Part model, mm, in its own coordinate system. A direction names the side the tool comes from. Round coordinates to 2 decimals unless told otherwise and drop trailing zeros. Loops run counter-clockwise (first coordinate to the right, second up) from the corner with the lowest first, then second, coordinate; pieces in that order, holes last. Notation, with made-up numbers: (-20.75, 76) - (24.25, 76) arc R24 cw to (24.25, 115) - close; hole circle Ø7 at (40, 48). An arc over 180 degrees is marked (long way). Put each result on its own line as item: value.
from build123d import *

# Parameters (mm, degrees)
SKETCH1_R           = 36
SKETCH1_R_2         = 13
BOSS_EXTRUDE1_DEPTH = 60
SKETCH2_W           = 9
SKETCH2_H           = 55


with BuildPart() as part:
    # Sketch1 → Boss-Extrude1 (new body)
    with BuildSketch(Plane(origin=(0, 0, 0), x_dir=(1, 0, 0), z_dir=(0, 1, 0))):
        Circle(SKETCH1_R)
        Circle(SKETCH1_R_2, mode=Mode.SUBTRACT)
    extrude(amount=BOSS_EXTRUDE1_DEPTH)

    # Sketch2 → Cut-Revolve1 (revolve, cut)
    with BuildSketch(Plane.XY):
        with Locations((-31.5, 30)):
            Rectangle(SKETCH2_W, SKETCH2_H)
    revolve(axis=Axis((0, 0, 0), (0, 1, 0)), mode=Mode.SUBTRACT)


solid = part.part
1. Band-saw the part on D-D (z = 23). List the corners of the cut face in (x, y).
A:
outline: (-27.69, 0) - (27.69, 0) - (27.69, 2.5) - (14.14, 2.5) - (14.14, 57.5) - (27.69, 57.5) - (27.69, 60) - (-27.69, 60) - (-27.69, 57.5) - (-14.14, 57.5) - (-14.14, 2.5) - (-27.69, 2.5) - close
2. Band-saw the part on C-C (y = 10). List the corners of the cut face in (x, z), plus the area to 3 significant figures.
A:
outline: circle Ø54 at (0, 0); hole circle Ø26 at (0, 0)
area: 1,760 mm²
3. Tool access for faces 1 (the flat face through (-5, 2.5, 27)), 2 (the cylindrical face through (-10.316, 29.58, 7.91)): list every direction of +Z, -Z, +X, -X, +Y, -Y with a clear straight run to the whole face (end or side of a thin tool).
A:
face 1: none
face 2: +Y, -Y
4. Two-plate mould, pull along Y, no slides. Class faces 3 (the flat face through (-1, 60, 15)), 4 (the flat face through (-5, 57.5, 27)), 5 (the cylindrical face through (-4.686, 1.232, -35.694)): pulls with the +Y half, pulls with the -Y half, needs draft (parallel to the pull), parting line crosses it, or undercut.
A:
face 3: pulls with the +Y half
face 4: undercut
face 5: needs draft
5. Pin check, flat tips, straight feed: P1, Ø12, axis at y = 45, z = -13.5, coming from the -X side; P2, Ø10, axis at x = -10.5, y = 43, coming from the -Z side; P3, Ø21.5, axis at x = 16.5, z = 10.5, coming from the -Y side; P4, Ø8, axis at y = 38, z = -13, coming from the -X side. Stop position of each tip, or through.
A:
P1: stops at x = -25.94
P2: stops at z = -26.43
P3: stops at y = 0
P4: stops at x = -25.46
6. Band-saw the part on B-B (z = 0). List the corners of the cut face in (x, y), plus the area to 3 significant figures.
A:
outline: (-36, 0) - (-13, 0) - (-13, 60) - (-36, 60) - (-36, 57.5) - (-27, 57.5) - (-27, 2.5) - (-36, 2.5) - close; (13, 0) - (36, 0) - (36, 2.5) - (27, 2.5) - (27, 57.5) - (36, 57.5) - (36, 60) - (13, 60) - close
area: 1,770 mm²
7. Band-saw the part on A-A (x = 0). List the corners of the cut face in (y, z), plus the area to 3 significant figures.
A:
outline: (0, -36) - (2.5, -36) - (2.5, -27) - (57.5, -27) - (57.5, -36) - (60, -36) - (60, -13) - (0, -13) - close; (0, 13) - (60, 13) - (60, 36) - (57.5, 36) - (57.5, 27) - (2.5, 27) - (2.5, 36) - (0, 36) - close
area: 1,770 mm²
8. Probe line 1 along Z through (x, y) = (0, 29); line 2 along Y through (x, z) = (-1, 32); line 3 along X through (y, z) = (26, -3). List the from-to ranges inside material, lowest first. Write a range as [from, to].
A:
line 1: z = [-27, -13], [13, 27]
line 2: y = [0, 2.5], [57.5, 60]
line 3: x = [-26.83, -12.65], [12.65, 26.83]
